```python
from build123d import *

# Parameters (mm, degrees)
SKETCH1_R               = 11.1
BOSS_EXTRUDE1_DEPTH     = 44.45
CUT_EXTRUDE1_REACH      = 82.845
SKETCH3_R               = 14.2875
CUT_EXTRUDE2_DEPTH      = 50.8
F_1_4_CLEARANCE_HOLE1_D = 7.14248
FILLET5_R               = 10.16


with BuildPart() as part:
    # Sketch1 → Boss-Extrude1 (new body)
    with BuildSketch(Plane(origin=(0, 0, 0), x_dir=(1, 0, 0), z_dir=(0, 1, 0))):
        with BuildLine():
            ThreePointArc((-47.655215915, -18.034), (-28.934565222, -7.31168908), (-7.858432995, -11.919005456))
            ThreePointArc((-7.858432995, -11.919005456), (14.27647226, 0), (-7.858432995, 11.919005456))
            ThreePointArc((-7.858432995, 11.919005456), (-28.934565222, 7.31168908), (-47.655215915, 18.034))
            Line((-47.655215915, 18.034), (-50.8, 18.034))
            Line((-50.8, 18.034), (-76.2, 18.034))
            Line((-76.2, 18.034), (-76.2, 12.954))
            Line((-76.2, 12.954), (-50.8, 12.954))
            Line((-50.8, 12.954), (-50.8, -12.954))
            Line((-50.8, -12.954), (-76.2, -12.954))
            Line((-76.2, -12.954), (-76.2, -18.034))
            Line((-76.2, -18.034), (-50.8, -18.034))
            Line((-50.8, -18.034), (-47.655215915, -18.034))
        make_face()
        with Locations(Location((0, 0, 0), (0, 0, 270))):
            Circle(SKETCH1_R, mode=Mode.SUBTRACT)
        with BuildLine():
            ThreePointArc((-46.99, -10.141749752), (-31.26726895, -2.566739092), (-13.840035745, -3.503008817))
            ThreePointArc((-13.840035745, -3.503008817), (-14.27647226, 0), (-13.840035745, 3.503008817))
            ThreePointArc((-13.840035745, 3.503008817), (-31.26726895, 2.566739092), (-46.99, 10.141749752))
            Line((-46.99, 10.141749752), (-46.99, -10.141749752))
        make_face(mode=Mode.SUBTRACT)
    extrude(amount=BOSS_EXTRUDE1_DEPTH)

    # Sketch2 → Cut-Extrude1 (cut, up to next)
    with BuildSketch(Plane.ZY.offset(50.8), mode=Mode.PRIVATE) as cut_extrude1_sk1:
        with BuildLine():
            Line((4.944497397, 33.298849711), (4.944497397, 11.151150289))
            ThreePointArc((4.944497397, 11.151150289), (0, 6.206652892), (-4.944497397, 11.151150289))
            Line((-4.944497397, 11.151150289), (-4.944497397, 33.298849711))
            ThreePointArc((-4.944497397, 33.298849711), (0, 38.243347108), (4.944497397, 33.298849711))
        make_face()
    cut_extrude1_tool1 = extrude(cut_extrude1_sk1.sketch, amount=-CUT_EXTRUDE1_REACH, mode=Mode.PRIVATE) & part.part
    add(cut_extrude1_tool1.solids().sort_by_distance((-50.8, 22.225, 0))[0], mode=Mode.SUBTRACT)

    # Sketch3 → Cut-Extrude2 (cut)
    with BuildSketch(Plane.XY.offset(18.034)):
        with Locations((-31.75, 22.225)):
            Circle(SKETCH3_R)
    extrude(amount=-CUT_EXTRUDE2_DEPTH, mode=Mode.SUBTRACT)

    # 1_4 Clearance Hole1 (through all)
    with Locations(Plane.XY.offset(18.034)):
        with Locations((-63.5, 35.687), (-63.5, 8.763)):
            Hole(F_1_4_CLEARANCE_HOLE1_D / 2)

    # Fillet5
    fillet5_edges = [part.edges().sort_by_distance(p)[0] for p in [
        (-76.2, 0, 15.494),
        (-76.2, 0, -15.494),
        (-76.2, 44.45, -15.494),
        (-76.2, 44.45, 15.494),
    ]]
    fillet(fillet5_edges, radius=FILLET5_R)


solid = part.part
```
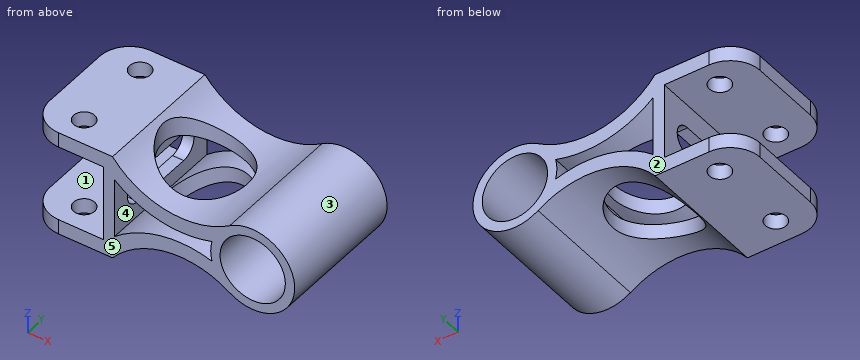
Verification items for the finished model (mm, model axes). Face numbers are marked on the shaded views. A direction names the side the tool comes from. Coordinates: 2 decimals unless noted, no trailing zeros. Order: outer loops, then holes, each group sorted by start corner. A loop starts at its lowest first (then second) coordinate and runs counter-clockwise, first axis right, second up. Notation, with made-up numbers: (15.25, -5) - (31.25, -5) arc R11 ccw to (31.25, 8) - close; hole circle Ø8 at (5.25, 74). An arc over 180 degrees is marked (long way). Return JSON: item names as keys, results as strings.
(1) Section check A-A, the plane x = 0. Record the cut outline in (y, z), and give its area (3 significant figures).
Filled sheet:
{"outline": "(0, -14.28) - (44.45, -14.28) - (44.45, -11.1) - (0, -11.1) - close; (0, 11.1) - (44.45, 11.1) - (44.45, 14.28) - (0, 14.28) - close", "area": "282 mm^2"}
(2) Section check C-C, the plane y = 15. Record the cut outline in (x, z).
Filled sheet:
{"outline": "(-76.2, -18.03) - (-47.66, -18.03) arc R30.01 cw to (-44.08, -14.33) - (-44.08, -7.93) arc R35.09 ccw to (-46.99, -10.14) - (-46.99, -4.94) - (-50.8, -4.94) - (-50.8, -12.95) - (-76.2, -12.95) - close; (-76.2, 12.95) - (-50.8, 12.95) - (-50.8, 4.94) - (-46.99, 4.94) - (-46.99, 10.14) arc R35.09 ccw to (-44.08, 7.93) - (-44.08, 14.33) arc R30.01 cw to (-47.66, 18.03) - (-76.2, 18.03) - close; (-19.42, -7.38) arc R30.01 cw to (-7.86, -11.92) arc R14.28 ccw (long way) to (-7.86, 11.92) arc R30.01 cw to (-19.42, 7.38) - (-19.42, 2.23) arc R35.09 ccw to (-13.84, 3.5) arc R14.28 ccw to (-13.84, -3.5) arc R35.09 ccw to (-19.42, -2.23) - close; hole circle Ø22.2 at (0, 0)"}
(3) Access from +Z, -Z, +X, -X, +Y, -Y to the whole of each face (thin tool, end or side, straight path). Record for the marked faces 1 and 2.
Filled sheet:
{"face 1": "-X, +Y, -Y", "face 2": "+Z, -Z, +X, -X, +Y"}
(4) Mould release check, pull along Z, two halves, no side actions. Record for the marked faces 3, 4 and 5: pulls with the +Z half, pulls with the -Z half, needs draft (parallel to the pull), parting line crosses it, or undercut.
Filled sheet:
{"face 3": "parting line crosses it", "face 4": "undercut", "face 5": "needs draft"}
(5) Section check D-D, the plane x = -63.5. Record the cut outline in (y, z), and give its area (3 significant figures).
Filled sheet:
{"outline": "(0, -18.03) - (5.19, -18.03) - (5.19, -12.95) - (0, -12.95) - close; (0, 12.95) - (5.19, 12.95) - (5.19, 18.03) - (0, 18.03) - close; (12.33, -18.03) - (32.12, -18.03) - (32.12, -12.95) - (12.33, -12.95) - close; (12.33, 12.95) - (32.12, 12.95) - (32.12, 18.03) - (12.33, 18.03) - close; (39.26, -18.03) - (44.45, -18.03) - (44.45, -12.95) - (39.26, -12.95) - close; (39.26, 12.95) - (44.45, 12.95) - (44.45, 18.03) - (39.26, 18.03) - close", "area": "306 mm^2"}
(6) Section check B-B, the plane z = 0. Record the cut outline in (x, y).
Filled sheet:
{"outline": "(-50.8, 0) - (-46.99, 0) - (-46.99, 6.21) - (-50.8, 6.21) - close; (-50.8, 38.24) - (-46.99, 38.24) - (-46.99, 44.45) - (-50.8, 44.45) - close; (-14.28, 0) - (-11.1, 0) - (-11.1, 44.45) - (-14.28, 44.45) - close; (11.1, 0) - (14.28, 0) - (14.28, 44.45) - (11.1, 44.45) - close"}
(7) Thickness scan on line 1 along Y through (x, z) = (-63.5, -15.7); line 2 along X through (y, z) = (40.5, 1); line 3 along X through (y, z) = (18, 10). Record the ranges inside material, lowest first.
Filled sheet:
{"line 1": "y = 0 to 5.19, 12.33 to 32.12, 39.26 to 44.45", "line 2": "x = -50.8 to -46.99, -14.24 to -11.05, 11.05 to 14.24", "line 3": "x = -50.8 to -46.99, -46.82 to -45.4, -11.22 to -4.82, 4.82 to 10.19"}
(8) Go/stop test with flat-tipped pins: pin 1 (5 mm diameter, centred on x = -19, y = 39, fed in from +Z); pin 2 (9.5 mm diameter, centred on x = -63.5, y = 8.763, fed in from +Z); pin 3 (23 mm diameter, centred on x = -31.75, y = 22.225, fed in from +Z); pin 4 (1 mm diameter, centred on y = 4.5, z = -0.5, fed in from -X). Record where each tip stops, or that it passes through.
Filled sheet:
{"pin 1": "stops at z = 8.02", "pin 2": "stops at z = 18.03", "pin 3": "passes through", "pin 4": "stops at x = -50.8"}
